Check sheet for the modelled part. Datum: model origin and axes. Units: mm. Face numbers are marked on the shaded views. Coordinates: 2 decimals unless noted, no trailing zeros. Loops run counter-clockwise (first coordinate to the right, second up) from the corner with the lowest first, then second, coordinate; pieces in that order, holes last. Notation, with made-up numbers: (13, -3.75) - (59, -3.75) arc R22 cw to (59, 2.25) - close; hole circle Ø1 at (-39.75, 30.25). An arc over 180 degrees is marked (long way). Write each question's results on one line, items separated by ' | '. Start each with the question number.
1. Cross-section at C-C (y = -36.5). Record the cut outline in (x, z), and give its area (3 significant figures).
2. Draft check along Z on the marked faces 1, 2 and 3. Enter one of: released by +Z, released by -Z, zero draft, split by the parting line, or undercut.
3. Gauge pin test, flat ends, axial feed: P1, Ø3, axis at x = 18, z = 144, coming from the -Y side; P2, Ø12, axis at x = -84.5, z = 162, coming from the +Y side; P3, Ø10, axis at x = -138.5, y = -15.5, coming from the +Z side. Record the tip position at first contact, or that the pin passes through.
4. Cross-section at A-A (x = -152.5). Record the cut outline in (y, z).
5. Cross-section at D-D (z = 157). Record the cut outline in (x, y), and give its area (3 significant figures).
6. Thickness scan on line 1 (Z direction, x = 100.5, y = -5.5); line 2 (Z direction, x = -119, y = -73.5); line 3 (Z direction, x = 114, y = -89). Record the ranges inside material, lowest first. Write a range as [from, to].
7. Cross-section at B-B (y = -122). Record the cut outline in (x, z), and give its area (3 significant figures).
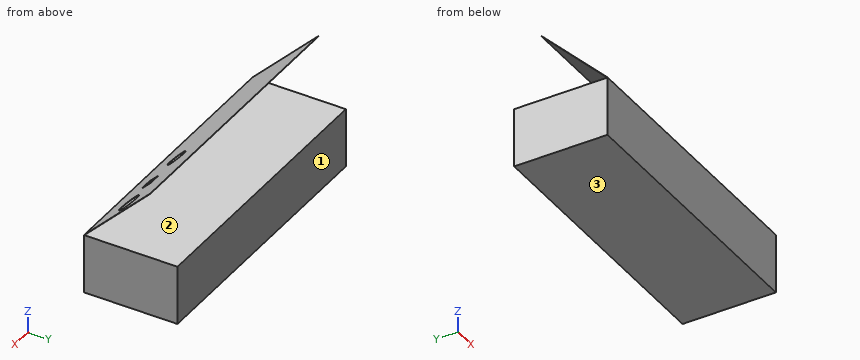
```python
from build123d import *

# Parameters (mm, degrees)
F1_DEPTH = 209.55
F3_DEPTH = 0.4064


# Not quite as in the source:
# - the dataset's text gives a spline's control points without its knots; the knots are read off the source's solid


with BuildPart() as f1:
    # F0 (on Right) → F1 (new body, symmetric)
    with BuildSketch(Plane.YZ):
        Polygon((-139.7, 0), (0, 0), (0, 88.9), (-139.2936, 88.9), (-139.2936, 89.154), (-40.6298144724, 187.8177855276), (-40.9171826682, 188.1051537235), (-139.7, 89.3223363917), align=None)
    extrude(amount=F1_DEPTH, both=True)

    # F2 (on face) → F3 (cut, through all)
    with BuildSketch(Plane(origin=(0, -114.5111681959, 114.5111681959), x_dir=(1, 0, 0), z_dir=(0, -0.7071067812, 0.7071067812))):
        with BuildLine():
            add(Edge.make_bspline(
                [(107.5209936486, 34.5596805655), (107.2271156486, 34.2660057655), (107.0557164486, 33.8529255655), (107.0557164486, 33.4373053655)],
                knots=[1, 1, 1, 1, 2, 2, 2, 2], degree=3))
            Line((107.0557164486, 33.4373053655), (107.0557164486, 16.7685553655))
            add(Edge.make_bspline(
                [(107.0557164486, 16.7685553655), (107.0557164486, 16.3530875655), (107.2271156486, 15.9400073655), (107.5209936486, 15.6461547655)],
                knots=[0, 0, 0, 0, 1, 1, 1, 1], degree=3))
            add(Edge.make_bspline(
                [(107.5209936486, 15.6461547655), (107.8148462486, 15.3522767655), (108.2279264486, 15.1810553655), (108.6432164486, 15.1810553655)],
                knots=[1, 1, 1, 1, 2, 2, 2, 2], degree=3))
            Line((108.6432164486, 15.1810553655), (125.3119664486, 15.1810553655))
            add(Edge.make_bspline(
                [(125.3119664486, 15.1810553655), (125.7282978486, 15.1810553655), (126.1410224486, 15.3522767655), (126.4352306486, 15.6461547655)],
                knots=[0, 0, 0, 0, 1, 1, 1, 1], degree=3))
            add(Edge.make_bspline(
                [(126.4352306486, 15.6461547655), (126.7287784486, 15.9400073655), (126.8994664486, 16.3530875655), (126.8994664486, 16.7685553655)],
                knots=[1, 1, 1, 1, 2, 2, 2, 2], degree=3))
            Line((126.8994664486, 16.7685553655), (126.8994664486, 33.4373053655))
            add(Edge.make_bspline(
                [(126.8994664486, 33.4373053655), (126.8994664486, 33.8529255655), (126.7287784486, 34.2660057655), (126.4352306486, 34.5596805655)],
                knots=[0, 0, 0, 0, 1, 1, 1, 1], degree=3))
            add(Edge.make_bspline(
                [(126.4352306486, 34.5596805655), (126.1410224486, 34.8537363655), (125.7282978486, 35.0248053655), (125.3119664486, 35.0248053655)],
                knots=[1, 1, 1, 1, 2, 2, 2, 2], degree=3))
            Line((125.3119664486, 35.0248053655), (108.6432164486, 35.0248053655))
            add(Edge.make_bspline(
                [(108.6432164486, 35.0248053655), (108.2279264486, 35.0248053655), (107.8148462486, 34.8537363655), (107.5209936486, 34.5596805655)],
                knots=[0, 0, 0, 0, 1, 1, 1, 1], degree=3))
        make_face()
        with BuildLine():
            add(Edge.make_bspline(
                [(67.0366194486, 40.2491027655), (64.3180828486, 42.9673091655), (60.4971608486, 44.5497799655), (56.6525914486, 44.5497799655)],
                knots=[7, 7, 7, 7, 8, 8, 8, 8], degree=3))
            add(Edge.make_bspline(
                [(56.6525914486, 44.5497799655), (52.8087078486, 44.5497799655), (48.9877858486, 42.9673091655), (46.2695794486, 40.2491027655)],
                knots=[0, 0, 0, 0, 1, 1, 1, 1], degree=3))
            add(Edge.make_bspline(
                [(46.2695794486, 40.2491027655), (43.5510936486, 37.5305661655), (41.9682164486, 33.7101267655), (41.9682164486, 29.8654303655), (41.9682164486, 26.0211911655), (43.5510936486, 22.2004469655), (46.2695794486, 19.4822405655)],
                knots=[1, 1, 1, 1, 2, 2, 2, 3, 3, 3, 3], degree=3))
            add(Edge.make_bspline(
                [(46.2695794486, 19.4822405655), (48.9877858486, 16.7637039655), (52.8087078486, 15.1810553655), (56.6525914486, 15.1810553655), (60.4971608486, 15.1810553655), (64.3180828486, 16.7637039655), (67.0366194486, 19.4822405655)],
                knots=[3, 3, 3, 3, 4, 4, 4, 5, 5, 5, 5], degree=3))
            add(Edge.make_bspline(
                [(67.0366194486, 19.4822405655), (69.7551814486, 22.2004469655), (71.3369664486, 26.0211911655), (71.3369664486, 29.8654303655), (71.3369664486, 33.7101267655), (69.7551814486, 37.5305661655), (67.0366194486, 40.2491027655)],
                knots=[5, 5, 5, 5, 6, 6, 6, 7, 7, 7, 7], degree=3))
        make_face()
        with BuildLine():
            add(Edge.make_bspline(
                [(189.0894868486, 43.6364975655), (186.0037170486, 46.7222673655), (181.6666416486, 48.5185299655), (177.3027692486, 48.5185299655)],
                knots=[7, 7, 7, 7, 8, 8, 8, 8], degree=3))
            add(Edge.make_bspline(
                [(177.3027692486, 48.5185299655), (172.9388714486, 48.5185299655), (168.6018468486, 46.7222673655), (165.5164072486, 43.6364975655)],
                knots=[0, 0, 0, 0, 1, 1, 1, 1], degree=3))
            add(Edge.make_bspline(
                [(165.5164072486, 43.6364975655), (162.4309930486, 40.5507277655), (160.6340192486, 36.2136777655), (160.6340192486, 31.8498053655), (160.6340192486, 27.4859075655), (162.4309930486, 23.1488575655), (165.5164072486, 20.0630877655)],
                knots=[1, 1, 1, 1, 2, 2, 2, 3, 3, 3, 3], degree=3))
            add(Edge.make_bspline(
                [(165.5164072486, 20.0630877655), (168.6018468486, 16.9776735655), (172.9388714486, 15.1810553655), (177.3027692486, 15.1810553655), (181.6666416486, 15.1810553655), (186.0037170486, 16.9776735655), (189.0894868486, 20.0630877655)],
                knots=[3, 3, 3, 3, 4, 4, 4, 5, 5, 5, 5], degree=3))
            add(Edge.make_bspline(
                [(189.0894868486, 20.0630877655), (192.1752312486, 23.1488575655), (193.9715192486, 27.4859075655), (193.9715192486, 31.8498053655), (193.9715192486, 36.2136777655), (192.1752312486, 40.5507277655), (189.0894868486, 43.6364975655)],
                knots=[5, 5, 5, 5, 6, 6, 6, 7, 7, 7, 7], degree=3))
        make_face()
    extrude(amount=-F3_DEPTH, mode=Mode.SUBTRACT)


solid = f1.part
```
Established:
1) outline: (-209.55, 0) - (209.55, 0) - (209.55, 88.9) - (-209.55, 88.9) - close | area: 37,300 mm^2
2) face 1: zero draft | face 2: undercut | face 3: released by -Z
3) P1: y = -86.52 | P2: y = -60.45 | P3: z = 88.9
4) outline: (-139.7, 0) - (0, 0) - (0, 88.9) - (-139.29, 88.9) - (-139.29, 89.15) - (-40.63, 187.82) - (-40.92, 188.11) - (-139.7, 89.32) - close
5) outline: (-209.55, -72.02) - (209.55, -72.02) - (209.55, -71.45) - (-209.55, -71.45) - close | area: 241 mm^2
6) line 1: [0, 88.9] | line 2: [0, 88.9], [154.95, 155.52] | line 3: [0, 88.9], [139.45, 140.02]
7) outline: (-209.55, 0) - (209.55, 0) - (209.55, 88.9) - (-209.55, 88.9) - close; (-209.55, 106.45) - (209.55, 106.45) - (209.55, 107.02) - (-209.55, 107.02) - close | area: 37,500 mm^2
